CAD build for the part. Positions are in the model's coordinates, mm. A direction names the side the tool comes from. Coordinates: 2 decimals unless noted, no trailing zeros. Loops run counter-clockwise (first coordinate to the right, second up) from the corner with the lowest first, then second, coordinate; pieces in that order, holes last.
1) Two-plate mould, pull along X, no slides. Class faces 4 (the flat face through (439.285, 74, 224)), 5 (the flat face through (273, 74, 374.071)), 6 (the flat face through (277, 81, 92.676)), 7 (the cylindrical face through (143.28, 80.98, 344.76)): +X half, -X half, draft (parallel to the pull), parting line (faces both ways), or undercut.
2) Wall check: line 1 along Z through (x, y) = (177.5, 114); line 2 along Z through (x, y) = (190, -249); line 3 along X through (y, z) = (-623, 478). Give the ranges that are in metal, low to high.
3) Which spindle directions (+Z, -Z, +X, -X, +Y, -Y) get a long thin tool onto all of the face, cutting with end or side? Do faces 1 (the cylindrical face through (425.027, 73.95, 85.383)), 2 (the flat face through (241.521, 210, 376)), 3 (the flat face through (419.54, 81, 226)). Say none if no direction does.
4) Saw through at B-B, the plane z = 224. Write the cut outline in (x, y).
5) Saw through at D-D, the plane y = -343. Write the cut outline in (x, z).
6) Saw through at C-C, the plane x = 58.5. Write the cut outline in (y, z), and give its area (3 significant figures).
7) Pin check, flat tips, straight feed: pin 1 Ø6 at (y, z) = (-647, 108.5) entering from +X; pin 2 Ø5 at (y, z) = (-530.5, -3.5) entering from -X; pin 3 Ø8 at (x, z) = (308.5, -6.5) entering from +Y. Stop position of each tip, or through.
8) Saw through at A-A, the plane y = 124.5. Write the cut outline in (x, z).
```python
from build123d import *

# Parameters (mm, degrees)
SKETCH_W      = 550
SKETCH_H      = 500
PAD_DEPTH     = 800
PAD001_DEPTH  = 150
POCKET_DEPTH  = 140
SKETCH003_R   = 33.237299
PAD002_DEPTH  = 200
PAD002_TAPER  = 2
SKETCH004_W   = 69.108994
SKETCH004_H   = 193.223083
PAD003_DEPTH  = 20
SKETCH005_W   = 517.289068
SKETCH005_H   = 25.703766
SKETCH005_W_2 = 488.372336
SKETCH005_H_2 = 22.490784
PAD004_DEPTH  = 10
SKETCH006_W   = 563.640388
SKETCH006_H   = 516.287299
PAD005_DEPTH  = 100


with BuildPart() as part:
    # Sketch → Pad (new body)
    with BuildSketch(Plane.XZ):
        with Locations((275, 250)):
            Rectangle(SKETCH_W, SKETCH_H)
    extrude(amount=PAD_DEPTH)

    # Sketch001 (on Face5 of Pad) → Pad001 (join)
    with BuildSketch(Plane(origin=(0, 0, 0), x_dir=(1, 0, 0), z_dir=(0, 1, 0))):
        with BuildLine():
            Line((110.821515, -120.347227), (110.821515, -324.071047))
            ThreePointArc((110.821515, -324.071047), (125.466176, -359.426386), (160.821515, -374.071047))
            Line((160.821515, -374.071047), (389.285222, -374.071047))
            ThreePointArc((389.285222, -374.071047), (424.640561, -359.426386), (439.285222, -324.071047))
            Line((439.285222, -324.071047), (439.285222, -120.347227))
            ThreePointArc((439.285222, -120.347227), (424.640561, -84.991888), (389.285222, -70.347227))
            Line((389.285222, -70.347227), (160.821515, -70.347227))
            ThreePointArc((160.821515, -70.347227), (125.466176, -84.991888), (110.821515, -120.347227))
        make_face()
    extrude(amount=PAD001_DEPTH)

    # Sketch002 (on Face15 of Pad001) → Pocket (cut)
    with BuildSketch(Plane(origin=(0, 150, 0), x_dir=(1, 0, 0), z_dir=(0, 1, 0))):
        with BuildLine():
            Line((131.86986, -132.675529), (131.86986, -316.786224))
            ThreePointArc((131.86986, -316.786224), (143.585589, -345.070495), (171.86986, -356.786224))
            Line((171.86986, -356.786224), (379.540297, -356.786224))
            ThreePointArc((379.540297, -356.786224), (407.824568, -345.070495), (419.540297, -316.786224))
            Line((419.540297, -316.786224), (419.540297, -132.675529))
            ThreePointArc((419.540297, -132.675529), (407.824568, -104.391258), (379.540297, -92.675529))
            Line((379.540297, -92.675529), (171.86986, -92.675529))
            ThreePointArc((171.86986, -92.675529), (143.585589, -104.391258), (131.86986, -132.675529))
        make_face()
    extrude(amount=-POCKET_DEPTH, mode=Mode.SUBTRACT)

    # Sketch003 (on Face4 of Pocket) → Pad002 (join)
    with BuildSketch(Plane(origin=(0, 0, 0), x_dir=(1, 0, 0), z_dir=(0, 1, 0))):
        with Locations((276.350006, -421.745483)):
            Circle(SKETCH003_R)
    extrude(amount=PAD002_DEPTH, taper=PAD002_TAPER)

    # Sketch004 (on Face17 of Pad002) → Pad003 (join)
    with BuildSketch(Plane(origin=(0, 200, 0), x_dir=(1, 0, 0), z_dir=(0, 1, 0))):
        with Locations((276.075752, -374.794769)):
            Rectangle(SKETCH004_W, SKETCH004_H)
    extrude(amount=PAD003_DEPTH)

    # Sketch005 (on Face1 of Pad003) → Pad004 (join)
    with BuildSketch(Plane(origin=(0, 0, 0), x_dir=(1, 0, 0), z_dir=(0, 0, -1))):
        with Locations((277.28729, 230.829208)):
            Rectangle(SKETCH005_W, SKETCH005_H)
        with Locations((272.467824, 524.816498)):
            Rectangle(SKETCH005_W_2, SKETCH005_H_2)
    extrude(amount=PAD004_DEPTH)

    # Sketch006 (on Face3 of Pad004) → Pad005 (join)
    with BuildSketch(Plane(origin=(0, 0, 0), x_dir=(1, 0, 0), z_dir=(0, 1, 0))):
        with Locations((275.736264, -248.714535)):
            Rectangle(SKETCH006_W, SKETCH006_H)
    extrude(amount=-PAD005_DEPTH)


solid = part.part
```
Data:
1. face 4: +X half
1. face 5: draft
1. face 6: undercut
1. face 7: undercut
2. line 1: z = 70.35 to 92.68, 356.79 to 374.07
2. line 2: z = 0 to 500
2. line 3: x = 0 to 550
3. face 1: -Z, +X, +Y
3. face 2: +Z, -Z, -X, +Y
3. face 3: +Y
4. outline: (-6.08, -100) - (0, -100) - (0, -800) - (550, -800) - (550, -100) - (557.56, -100) - (557.56, 0) - (439.29, 0) - (439.29, 150) - (419.54, 150) - (419.54, 10) - (131.87, 10) - (131.87, 150) - (110.82, 150) - (110.82, 0) - (-6.08, 0) - close
5. outline: (0, 0) - (550, 0) - (550, 500) - (0, 500) - close
6. outline: (-800, 0) - (-536.06, 0) - (-536.06, -10) - (-513.57, -10) - (-513.57, 0) - (-243.68, 0) - (-243.68, -10) - (-217.98, -10) - (-217.98, 0) - (-100, 0) - (-100, -9.43) - (0, -9.43) - (0, 506.86) - (-100, 506.86) - (-100, 500) - (-800, 500) - close
6. area: 402,000 mm2
7. pin 1: stops at x = 550
7. pin 2: stops at x = 28.28
7. pin 3: stops at y = 0
8. outline: (110.82, 120.35) arc R50 ccw to (160.82, 70.35) - (389.29, 70.35) arc R50 ccw to (439.29, 120.35) - (439.29, 324.07) arc R50 ccw to (389.29, 374.07) - (160.82, 374.07) arc R50 ccw to (110.82, 324.07) - close; circle Ø57.78 at (276.35, 421.75); hole (131.87, 132.68) arc R40 ccw to (171.87, 92.68) - (379.54, 92.68) arc R40 ccw to (419.54, 132.68) - (419.54, 316.79) arc R40 ccw to (379.54, 356.79) - (171.87, 356.79) arc R40 ccw to (131.87, 316.79) - close
